Autodesk Inventor part; units mm, degrees
ref_plane "YZ Plane" through (0, 0, 0) normal (1, 0, 0) x (0, 1, 0)
ref_plane "XZ Plane" through (0, 0, 0) normal (0, 1, 0) x (-1, 0, 0)
ref_plane "XY Plane" through (0, 0, 0) normal (0, 0, 1) x (1, 0, 0)
sketch "Sketch1" plane through (0, 0, 0) normal (0, 0, 1) x (1, 0, 0)
  line L0 (-8.9346, 3.531) -> (-24.9346, 3.531)
  line L1 (-24.9346, 3.531) -> (-24.9346, 45.531)
  line L2 (-24.9346, 45.531) -> (17.0654, 45.531)
  line L3 (17.0654, 45.531) -> (17.0654, 3.531)
  line L4 (17.0654, 3.531) -> (1.0654, 3.531)
  line L5 (4.0654, 27.1063) -> (2.3055, 18.8848)
  line L6 (2.3055, 18.8848) -> (-5.6945, 16.2981)
  line L7 (-5.6945, 16.2981) -> (-11.9346, 21.933)
  line L8 (-11.9346, 21.933) -> (-10.1748, 30.1545)
  line L9 (-10.1748, 30.1545) -> (-2.1748, 32.7412)
  line L10 (-2.1748, 32.7412) -> (4.0654, 27.1063)
  circle A0 centre (-3.9346, 24.5196) radius 3.5
  line L11 (-8.9346, -0.469) -> (1.0654, -0.469)
  line L12 (-8.9346, 3.531) -> (-8.9346, -0.469)
  line L13 (1.0654, 3.531) -> (1.0654, -0.469)
  point P0 (0, 0)
extrude "Extrusion1" add sketch "Sketch1" against normal blind 10 contours L0 L1 L2 L3 L4 L13 L11 L12 | L5 L6 L7 L8 L9 L10 | A0
extrude "Extrusion2" cut sketch "Sketch1" against normal through all contours A0
extrude "Extrusion3" cut sketch "Sketch1" against normal blind 5 contours L5 L6 L7 L8 L9 L10
sketch "Sketch2" plane through (-24.9346, 45.531, 0) normal (0, 1, 0) x (1, 0, 0)
  line L0 (3.5162, 3.5162) -> (38.4838, 3.5162)
  line L1 (38.4838, 3.5162) -> (38.4838, 6.4838)
  line L2 (38.4838, 6.4838) -> (3.5162, 6.4838)
  line L3 (3.5162, 6.4838) -> (3.5162, 3.5162)
  point P0 (24.9346, 0)
  point P1 (0, 10)
  point P2 (42, 0)
extrude "Extrusion4" cut sketch "Sketch2" against normal blind 10
properties part number "gaica cu suportul" material "Gold"
Verification items for the finished model (mm, model axes). A direction names the side the tool comes from. Coordinates: 2 decimals unless noted, no trailing zeros. Loops run counter-clockwise (first coordinate to the right, second up) from the corner with the lowest first, then second, coordinate; pieces in that order, holes last. Notation, with made-up numbers: (-6.75, 16.25) -> (19.25, 16.25) arc R27 cw to (19.25, 36.25) -> close; hole circle Ø11 at (89, 70). An arc over 180 degrees is marked (long way). Answer in a Markdown table with one row per item. Add a question column.
1. Depth check by flat-ended pin: P1, Ø5, axis at x = 12.5, z = -2.5, coming from the -Y side; P2, Ø4.5, axis at y = 1, z = -6, coming from the -X side; P3, Ø1.5, axis at x = -6, z = -5, coming from the +Y side; P4, Ø5.5, axis at x = -3.93, y = 24.52, coming from the -Z side. Enter the tip coordinate at first touch or a pass-through.
2. Section check B-B, the plane z = -1.5. Enter the section's corners in (x, y).
3. Section check C-C, the plane x = 11. Enter the section's corners in (y, z).
4. Section check A-A, the plane y = 38.5. Enter the section's corners in (x, z), then the cut area to 3 significant figures.
5. Access from +Z, -Z, +X, -X, +Y, -Y to the whole of each face (thin tool, end or side, straight path). Record for faces 1 (the face through (-8.935, 2, -5)), 2 (the face through (9, 3.531, -5)), 3 (the face through (-8.8, 19.1, -2.5)), 4 (the face through (-4, 41, -3.516)).
6. Material ranges on probe 1 along Z at (x, y) = (-3, 17.5); probe 2 along Z at (x, y) = (0.5, 38.5); probe 3 along X at (y, z) = (3, -6.5), recorded low to high. Write a range as [from, to].
7. Section check D-D, the plane y = 3. Enter the section's corners in (x, z), then the cut area to 3 significant figures.
8. Draft check along X on faces 5 (the face through (3.198, 23.053, -2.465)), 6 (the face through (-4, 45.531, -3)), 7 (the face through (1.065, 2, -5)). Enter one of: +X half, -X half, draft (parallel to the pull), parting line (faces both ways), or undercut.
Derived:
| question | item | result |
|---|---|---|
| 1 | P1 | stops at y = 3.53 |
| 1 | P2 | stops at x = -8.93 |
| 1 | P3 | stops at y = 35.53 |
| 1 | P4 | passes through |
| 2 | outline | (-24.93, 3.53) -> (-8.93, 3.53) -> (-8.93, -0.47) -> (1.07, -0.47) -> (1.07, 3.53) -> (17.07, 3.53) -> (17.07, 45.53) -> (-24.93, 45.53) -> close; hole (-11.93, 21.93) -> (-5.69, 16.3) -> (2.31, 18.88) -> (4.07, 27.11) -> (-2.17, 32.74) -> (-10.17, 30.15) -> close |
| 3 | outline | (3.53, -10) -> (45.53, -10) -> (45.53, -6.48) -> (35.53, -6.48) -> (35.53, -3.52) -> (45.53, -3.52) -> (45.53, 0) -> (3.53, 0) -> close |
| 4 | outline | (-24.93, -10) -> (17.07, -10) -> (17.07, 0) -> (-24.93, 0) -> close; hole (-21.42, -6.48) -> (13.55, -6.48) -> (13.55, -3.52) -> (-21.42, -3.52) -> close |
| 4 | area | 316 mm² |
| 5 | face 1 | +Z, -Z, -X, -Y |
| 5 | face 2 | +Z, -Z, +X, -Y |
| 5 | face 3 | +Z |
| 5 | face 4 | +Y |
| 6 | probe 1 | z = [-10, -5] |
| 6 | probe 2 | z = [-10, -6.48], [-3.52, 0] |
| 6 | probe 3 | x = [-8.93, 1.07] |
| 7 | outline | (-8.93, -10) -> (1.07, -10) -> (1.07, 0) -> (-8.93, 0) -> close |
| 7 | area | 100 mm² |
| 8 | face 5 | undercut |
| 8 | face 6 | draft |
| 8 | face 7 | +X half |
